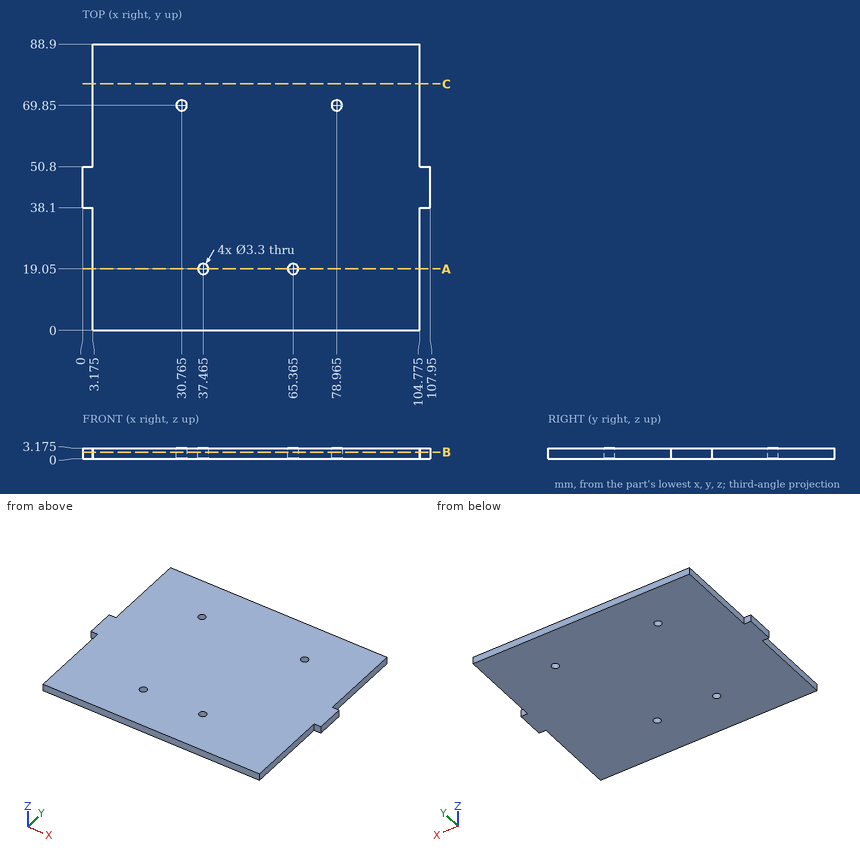
Study the drawing (mm; zero at the part's minimum x, y, z) and answer. Round coordinates to 2 decimals unless told otherwise and drop trailing zeros. Write each loop counter-clockwise with the first axis right and the second up, starting at its lowest first coordinate (ties: lowest second). Pieces come first, ordered by that corner, then holes. Notation, with made-up numbers: (21.25, 68.25) - (37.25, 68.25) arc R15 ccw to (37.25, 88.25) - close; hole circle Ø11 at (69.5, 86). An arc over 180 degrees is marked (long way). Return JSON: item names as keys, results as strings. Group by question number.
Q1. The part is cut by section C-C on y = 76.5. Write down the section's boundary in (x, z) (3 decimals).
Q2. Each of these flat-tipped pins is pushed along its axis until it touches: pin 1 Ø4 at (x, y) = (37.465, 19.05) entering from -Z; pin 2 Ø1.6 at (x, z) = (1.5, 1) entering from -Y. Where does it stop, or does it pass through?
Q3. The part is cut by section A-A on y = 19.05. Write down the section's boundary in (x, z) (3 decimals), then the cut area to 3 significant figures.
Q4. The part is cut by section B-B on z = 2. Write down the section's boundary in (x, y) (3 decimals).
Q5. Find the intervals of material crossed by L1, parallel to X at y = 69.85, z = 1.85 (3 decimals); L2, parallel to X at y = 35, z = 0.1 (3 decimals); L3, parallel to Y at x = 37, z = 2.15, in increasing order.
Solved:
{
 "1": {"outline": "(3.175, 0) - (104.775, 0) - (104.775, 3.175) - (3.175, 3.175) - close"},
 "2": {"pin 1": "z = 0", "pin 2": "y = 38.1"},
 "3": {"outline": "(3.175, 0) - (35.815, 0) - (35.815, 3.175) - (3.175, 3.175) - close; (39.115, 0) - (63.715, 0) - (63.715, 3.175) - (39.115, 3.175) - close; (67.015, 0) - (104.775, 0) - (104.775, 3.175) - (67.015, 3.175) - close", "area": "302 mm²"},
 "4": {"outline": "(0, 38.1) - (3.175, 38.1) - (3.175, 0) - (104.775, 0) - (104.775, 38.1) - (107.95, 38.1) - (107.95, 50.8) - (104.775, 50.8) - (104.775, 88.9) - (3.175, 88.9) - (3.175, 50.8) - (0, 50.8) - close; hole circle Ø3.3 at (30.765, 69.85); hole circle Ø3.3 at (37.465, 19.05); hole circle Ø3.3 at (65.365, 19.05); hole circle Ø3.3 at (78.965, 69.85)"},
 "5": {"L1": "3.175 to 29.115, 32.415 to 77.315, 80.615 to 104.775", "L2": "3.175 to 104.775", "L3": "0 to 17.47, 20.63 to 88.9"}
}
